```python
from build123d import *

# Parameters (mm, degrees)
BOSS_EXTRUDE1_DEPTH                        = 40
CUT_EXTRUDE2_DEPTH                         = 25
CUT_EXTRUDE4_DEPTH                         = 208.846096908
F_2_0MM_DOWEL_HOLE1_D                      = 2
F_2_0MM_DOWEL_HOLE1_DEPTH                  = 9
F_2_0MM_DOWEL_HOLE1_CSINK_D                = 2.05
F_2_0MM_DOWEL_HOLE1_CSINK_ANGLE            = 90
F_2_0MM_DOWEL_HOLE1_TIP                    = 0.600860619
SKETCH11_W                                 = 23.5
SKETCH11_H                                 = 12
CUT_EXTRUDE3_DEPTH                         = 206.48722588
FILLET7_R                                  = 5
FILLET6_R                                  = 2
CBORE_FOR_M5_CHEESE_HEAD_SCREW1_AT_2_COUNT = 2
CBORE_FOR_M5_CHEESE_HEAD_SCREW1_AT_2_PITCH = 36
CBORE_FOR_M5_CHEESE_HEAD_SCREW1_AT_3_COUNT = 2
CBORE_FOR_M5_CHEESE_HEAD_SCREW1_AT_3_PITCH = 30
CBORE_FOR_M5_CHEESE_HEAD_SCREW1_AT_4_COUNT = 2
CBORE_FOR_M5_CHEESE_HEAD_SCREW1_AT_4_PITCH = 46.861498055
FILLET8_R                                  = 20


with BuildPart() as part:
    # Sketch1 → Boss-Extrude1 (new body)
    with BuildSketch(Plane.XY):
        Polygon((0, 0), (-200, 0), (-200, 40), (-50, 40), (-50, 9), (0, 9), align=None)
    extrude(amount=BOSS_EXTRUDE1_DEPTH)

    # Sketch5 → Cut-Extrude2 (cut)
    with BuildSketch(Plane.XY.offset(40)):
        Polygon((-145, 40), (-160, 31.339745962), (-160, 8.660254038), (-145, 0), (-200, 0), (-200, 40), align=None)
    extrude(amount=-CUT_EXTRUDE2_DEPTH, mode=Mode.SUBTRACT)

    # Sketch13 → Cut-Extrude4 (cut, through all)
    with BuildSketch(Plane.XY.offset(40)):
        Polygon((-50, 31.339745962), (-65, 40), (-50, 40), align=None)
    extrude(amount=-CUT_EXTRUDE4_DEPTH, mode=Mode.SUBTRACT)

    # Ø2.0mm Dowel Hole1
    with Locations(Plane.XY.offset(15)):
        with Locations((-194.2, 19.664446974), (-165.8, 19.664446974)):
            CounterSinkHole(F_2_0MM_DOWEL_HOLE1_D / 2, F_2_0MM_DOWEL_HOLE1_CSINK_D / 2, depth=F_2_0MM_DOWEL_HOLE1_DEPTH, counter_sink_angle=F_2_0MM_DOWEL_HOLE1_CSINK_ANGLE)
            with Locations((0, 0, -(F_2_0MM_DOWEL_HOLE1_DEPTH + F_2_0MM_DOWEL_HOLE1_TIP / 2))):  # 118° drill point
                Cone(0, F_2_0MM_DOWEL_HOLE1_D / 2, F_2_0MM_DOWEL_HOLE1_TIP, mode=Mode.SUBTRACT)

    # Sketch11 → Cut-Extrude3 (cut, through all)
    with BuildSketch(Plane.XY.offset(15)):
        with Locations((-180, 19.664446974)):
            Rectangle(SKETCH11_W, SKETCH11_H)
    extrude(amount=-CUT_EXTRUDE3_DEPTH, mode=Mode.SUBTRACT)

    # Fillet7
    fillet7_edges = [part.edges().sort_by_distance(p)[0] for p in [
        (-145, 40, 27.5),
        (-160, 31.339745962, 27.5),
        (-160, 8.660254038, 27.5),
        (-50, 31.339745962, 20),
        (-65, 40, 20),
    ]]
    fillet(fillet7_edges, radius=FILLET7_R)

    # Fillet6
    fillet6_edges = [part.edges().sort_by_distance(p)[0] for p in [
        (-50, 18.726497308, 40),
        (-151.25, 3.608439182, 40),
        (-58.169872981, 36.056624327, 40),
        (-105, 40, 40),
        (-151.830127019, 36.056624327, 40),
        (-160, 20, 40),
        (-159.330127019, 30.952994616, 40),
        (-159.330127019, 9.047005384, 40),
        (-144.954349263, 39.829629131, 40),
        (-50.669872981, 30.952994616, 40),
        (-65.045650737, 39.829629131, 40),
    ]]
    fillet(fillet6_edges, radius=FILLET6_R)

    # Sketch3 → CBORE for M5 Cheese Head Screw1 (revolve, cut)
    with BuildSketch(Plane(origin=(-43, 9, 5), x_dir=(0, 0, 1), z_dir=(1, 0, 0))):
        Polygon((0, 0), (0, 9), (1.7, 9), (1.7, 3), (3.25, 3), (3.25, 1.525), (4.775, 0), align=None)
    cbore_for_m5_cheese_head_screw1 = revolve(axis=Axis((-43, 15.35, 5), (0, -1, 0)), mode=Mode.SUBTRACT)

    # CBORE for M5 Cheese Head Screw1 at 2: CBORE for M5 Cheese Head Screw1 ×2
    with Locations(*[(i * CBORE_FOR_M5_CHEESE_HEAD_SCREW1_AT_2_PITCH, 0, 0) for i in range(1, CBORE_FOR_M5_CHEESE_HEAD_SCREW1_AT_2_COUNT)]):
        add(cbore_for_m5_cheese_head_screw1, mode=Mode.SUBTRACT)

    # CBORE for M5 Cheese Head Screw1 at 3: CBORE for M5 Cheese Head Screw1 ×2
    with Locations(*[(0, 0, i * CBORE_FOR_M5_CHEESE_HEAD_SCREW1_AT_3_PITCH) for i in range(1, CBORE_FOR_M5_CHEESE_HEAD_SCREW1_AT_3_COUNT)]):
        add(cbore_for_m5_cheese_head_screw1, mode=Mode.SUBTRACT)

    # CBORE for M5 Cheese Head Screw1 at 4: CBORE for M5 Cheese Head Screw1 ×2
    with Locations(*[Vector(0.7682212795973759, 0, 0.6401843996644799) * (i * CBORE_FOR_M5_CHEESE_HEAD_SCREW1_AT_4_PITCH) for i in range(1, CBORE_FOR_M5_CHEESE_HEAD_SCREW1_AT_4_COUNT)]):
        add(cbore_for_m5_cheese_head_screw1, mode=Mode.SUBTRACT)

    # Fillet8
    fillet8_edges = [part.edges().sort_by_distance(p)[0] for p in [
        (-200, 0, 7.5),
        (-200, 40, 7.5),
    ]]
    fillet(fillet8_edges, radius=FILLET8_R - 0.0001)  # a hair under: the kernel refuses the full size


solid = part.part
```
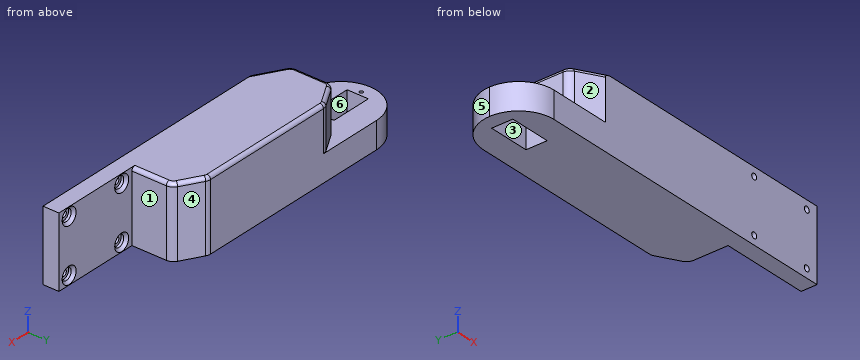
Geometry check sheet. Reference: the model listing, model coordinates, mm. Face numbers are marked on the shaded views. A direction names the side the tool comes from. Give positions to 0.01 mm unless a question says otherwise; leave off trailing zeros. Loops run counter-clockwise (first coordinate to the right, second up) from the corner with the lowest first, then second, coordinate; pieces in that order, holes last. Notation, with made-up numbers: M 65,72 L 74,72 A12 ccw 74,77 Z; hole C 82.5,-20.75 d10. An arc over 180 degrees is marked long. Write item = value, one per line.
(1) Sectioned sample at C-C, the plane y = 23. Record the cut outline in (x, z), plus the area to 3 significant figures.
Answer below:
outline = M -199.77,0 L -191.75,0 L -191.75,15 L -199.77,15 Z; M -168.25,0 L -50,0 L -50,38 A2 ccw -52,40 L -158,40 A2 ccw -160,38 L -160,15 L -168.25,15 Z
area = 4,640 mm2
(2) Sectioned sample at D-D, the plane z = 24.5. Record the cut outline in (x, y), plus the area to 3 significant figures.
Answer below:
outline = M -160,11.55 A5 ccw -157.5,7.22 L -145,0 L 0,0 L 0,9 L -50,9 L -50,28.45 A5 ccw -52.5,32.78 L -63.84,39.33 A5 ccw -66.34,40 L -143.66,40 A5 ccw -146.16,39.33 L -157.5,32.78 A5 ccw -160,28.45 Z
area = 4,650 mm2
(3) Gauge pin test, flat ends, axial feed: pin 1 Ø7.5 at (x, z) = (-7, 5) entering from -Y; pin 2 Ø12 at (x, z) = (-31.5, 26.5) entering from +Y; pin 3 Ø4 at (y, z) = (10, 36) entering from -X; pin 4 Ø6 at (y, z) = (32, 12) entering from -X. Record the tip position at first contact, or that the pin passes through.
Answer below:
pin_1 = 0
pin_2 = 9
pin_3 = -160
pin_4 = -197.86
(4) Tool access check on the marked faces 1, 2 and 3. Record the directions out of +Z, -Z, +X, -X, +Y, -Y that give a thin tool (end or side, any length) a straight path to the whole face; none if there is none.
Answer below:
face_1 = +Z, -Z, +X, +Y
face_2 = +Z, -X, -Y
face_3 = +Z, -Z
(5) Sectioned sample at B-B, the plane x = -43. Record the cut outline in (y, z) (3 decimals).
Answer below:
outline = M 0,0 L 9,0 L 9,0.225 L 7.475,1.75 L 6,1.75 L 6,3.3 L 0,3.3 Z; M 0,6.7 L 6,6.7 L 6,8.25 L 7.475,8.25 L 9,9.775 L 9,30.225 L 7.475,31.75 L 6,31.75 L 6,33.3 L 0,33.3 Z; M 0,36.7 L 6,36.7 L 6,38.25 L 7.475,38.25 L 9,39.775 L 9,40 L 0,40 Z
(6) Material ranges on line 1 (Z direction, x = -43, y = 6.9); line 2 (Z direction, x = -43, y = 3.45); line 3 (X direction, y = 8.5, z = 8), recorded low to high. Write a range as [from, to].
Answer below:
line_1 = [0, 1.75], [8.25, 31.75], [38.25, 40]
line_2 = [0, 3.3], [6.7, 33.3], [36.7, 40]
line_3 = [-196.36, -46.05], [-39.95, -10.05], [-3.95, 0]
(7) Sectioned sample at A-A, the plane z = 35. State how many separate pieces and enclosed holes the cut face has, plus the area to 3 significant figures.
Answer below:
separate_pieces = 3
enclosed_holes = 0
area = 4,570 mm2
(8) Release check for a two-part mould opening along X. For the marked faces 4, 5 and 6 record: released by +X, released by -X, zero draft, split by the parting line, or undercut.
Answer below:
face_4 = released by +X
face_5 = released by -X
face_6 = undercut
